from build123d import *

# Parameters (mm, degrees)
SKETCH2_R           = 11
BOSS_EXTRUDE1_DEPTH = 1
BOSS_EXTRUDE2_START = 8
SKETCH3_R           = 11
SKETCH3_R_2         = 8
BOSS_EXTRUDE2_DEPTH = 8
SKETCH4_R           = 8
CUT_EXTRUDE1_DEPTH  = 34.496268449
SKETCH5_W           = 1.5
SKETCH5_H           = 6.215499562
CIRPATTERN1_COUNT   = 3


with BuildPart() as part:
    # Sketch1 → Revolve1 (revolve)
    with BuildSketch(Plane.XY, mode=Mode.PRIVATE) as revolve1_sk:
        Polygon((0, 0), (0, 21), (5, 21), (5, 23), (6, 23), (6, 0), align=None)
    revolve(revolve1_sk.sketch.rotate(Axis((0, 0, 0), (1, 0, 0)), 90), axis=Axis((0, 0, 0), (1, 0, 0)))

    # Sketch2 → Boss-Extrude1 (add)
    with BuildSketch(Plane(origin=(6, 0, 0), x_dir=(0, 0, -1), z_dir=(1, 0, 0))):
        with Locations((0, -10)):
            Circle(SKETCH2_R)
    extrude(amount=BOSS_EXTRUDE1_DEPTH)

    # Sketch3 → Boss-Extrude2 (add)
    with BuildSketch(Plane.ZY.offset(BOSS_EXTRUDE2_START)):
        with Locations(Location((0, -10, 0), (0, 0, 180))):
            Circle(SKETCH3_R)
        with Locations((0, -10)):
            Circle(SKETCH3_R_2, mode=Mode.SUBTRACT)
    extrude(amount=-BOSS_EXTRUDE2_DEPTH)

    # Sketch4 → Cut-Extrude1 (cut, through all)
    with BuildSketch(Plane.ZY):
        with Locations((0, -10)):
            Circle(SKETCH4_R)
    extrude(amount=-CUT_EXTRUDE1_DEPTH, mode=Mode.SUBTRACT)

    # Sketch5 → Cut-Revolve3 (revolve, cut)
    with BuildSketch(Plane.XY, mode=Mode.PRIVATE) as cut_revolve3_sk:
        with Locations((-4.75, -19.69259974)):
            Rectangle(SKETCH5_W, SKETCH5_H)
    cut_revolve3 = revolve(cut_revolve3_sk.sketch.rotate(Axis((-4, -21, 0), (0, 1, 0)), 270), axis=Axis((-4, -21, 0), (0, 1, 0)), mode=Mode.SUBTRACT)

    # CirPattern1: Cut-Revolve3 ×3 about axis
    cirpattern1_axis = Axis((-8, -10, 0), (1, 0, 0))
    for i in range(1, CIRPATTERN1_COUNT):
        add(cut_revolve3.rotate(cirpattern1_axis, i * 360 / CIRPATTERN1_COUNT), mode=Mode.SUBTRACT)


solid = part.part
Design review of the part built by this model. Coordinates are the model's own, in mm. A direction names the side the tool comes from. Coordinates: 2 decimals unless noted, no trailing zeros. Write each loop counter-clockwise with the first axis right and the second up, starting at its lowest first coordinate (ties: lowest second). Pieces come first, ordered by that corner, then holes. Notation, with made-up numbers: (-30.75, 81.5) - (-11.75, 81.5) arc R23 ccw to (-11.75, 100.5) - close; hole circle Ø11 at (-17, 23). An arc over 180 degrees is marked (long way). One line per item, written item: value.
1) Add section B-B (z = 4.5). State the section outline as (x, y) points.
Answer sheet:
outline: (-8, -20.04) - (0, -20.04) - (0, -20.51) - (5, -20.51) - (5, -22.56) - (6, -22.56) - (6, -20.04) - (7, -20.04) - (7, -16.61) - (-8, -16.61) - close; (-8, -3.39) - (7, -3.39) - (7, 0.04) - (6, 0.04) - (6, 22.56) - (5, 22.56) - (5, 20.51) - (0, 20.51) - (0, 0.04) - (-8, 0.04) - close
2) Insertion check: pin 1 (1.5 mm diameter, centred on y = 13.5, z = 0, fed in from -X); pin 2 (14.5 mm diameter, centred on y = -10, z = 0, fed in from +X); pin 3 (2.5 mm diameter, centred on x = -4, z = 0, fed in from -Y); pin 4 (4 mm diameter, centred on x = 1.5, z = -1.5, fed in from -Y). Each pin has a flat end and moves straight along its axis. Give the tip position at first contact, or say it passes through.
Answer sheet:
pin 1: stops at x = 0
pin 2: passes through
pin 3: stops at y = -2.1
pin 4: stops at y = -21
3) Add section D-D (x = -6.5). State the section outline as (y, z) points, plus the area to 3 significant figures.
Answer sheet:
outline: circle Ø22 at (-10, 0); hole circle Ø16 at (-10, 0)
area: 179 mm2
4) Add section C-C (y = -10). State the section outline as (x, z) points, plus the area to 3 significant figures.
Answer sheet:
outline: (-8, -11) - (0, -11) - (0, -18.47) - (5, -18.47) - (5, -20.71) - (6, -20.71) - (6, -11) - (7, -11) - (7, -8) - (-8, -8) - close; (-8, 8) - (7, 8) - (7, 11) - (6, 11) - (6, 20.71) - (5, 20.71) - (5, 18.47) - (0, 18.47) - (0, 11) - (-8, 11) - close
area: 184 mm2
5) For faces 5 (the face through (-5.265, -19.407, -0.806)), 6 (the face through (5, 19, -10)), 7 (the face through (-8, -2, 2)), list the 3-axis set-ups (+Z, -Z, +X, -X, +Y, -Y) from which the entire face can be reached by the end or side of a thin tool; tool diameter is ignored.
Answer sheet:
face 5: -Y
face 6: -X
face 7: +Z, -Z, -X, +Y, -Y
6) Add section A-A (x = -4). State the section outline as (y, z) points.
Answer sheet:
outline: (-20.9, -1.5) arc R11 ccw to (-5.85, -10.19) - (-7.37, -7.56) arc R8 cw to (-17.86, -1.5) - close; (-20.9, 1.5) - (-17.86, 1.5) arc R8 cw to (-7.37, 7.56) - (-5.85, 10.19) arc R11 ccw to start; (-4.77, -6.06) - (-3.25, -8.69) arc R11 ccw to (-3.25, 8.69) - (-4.77, 6.06) arc R8 cw to start
7) Mouldability with a two-part tool opening along Y and no side actions: class faces 1 (the face through (6.49, -20.74, 2.38)), 2 (the face through (7, -18, 2)), 3 (the face through (-0.61, -17.81, -1.73)), 4 (the face through (-4.451, -6.536, 8.862)) as +Y half, -Y half, draft (parallel to the pull), parting line (faces both ways), or undercut.
Answer sheet:
face 1: parting line
face 2: draft
face 3: undercut
face 4: undercut
8) To check wall thickness, follow probe 1 along X at (y, z) = (-20.15, 0); probe 2 along Y at (x, z) = (3.25, 0); probe 3 along Y at (x, z) = (-1.5, 0). State the ranges of each line that lie inside material, in increasing order.
Answer sheet:
probe 1: x = -8 to -5.5, -2.5 to 7
probe 2: y = -21 to -18, -2 to 21
probe 3: y = -21 to -18, -2 to 1
